The figure shows three views and two pictorial views of one solid part (mm, origin at its lowest corner). Answer the questions. A direction names the side the tool comes from. Coordinates: 2 decimals unless noted, no trailing zeros. Write each loop counter-clockwise with the first axis right and the second up, starting at its lowest first coordinate (ties: lowest second). Pieces come first, ordered by that corner, then holes. Notation, with made-up numbers: M -37,87.25 L -28,87.25 A15 cw -28,100.25 Z; hole C -22,9.25 d8. An arc over 180 degrees is marked long. Write item = value, one per line.
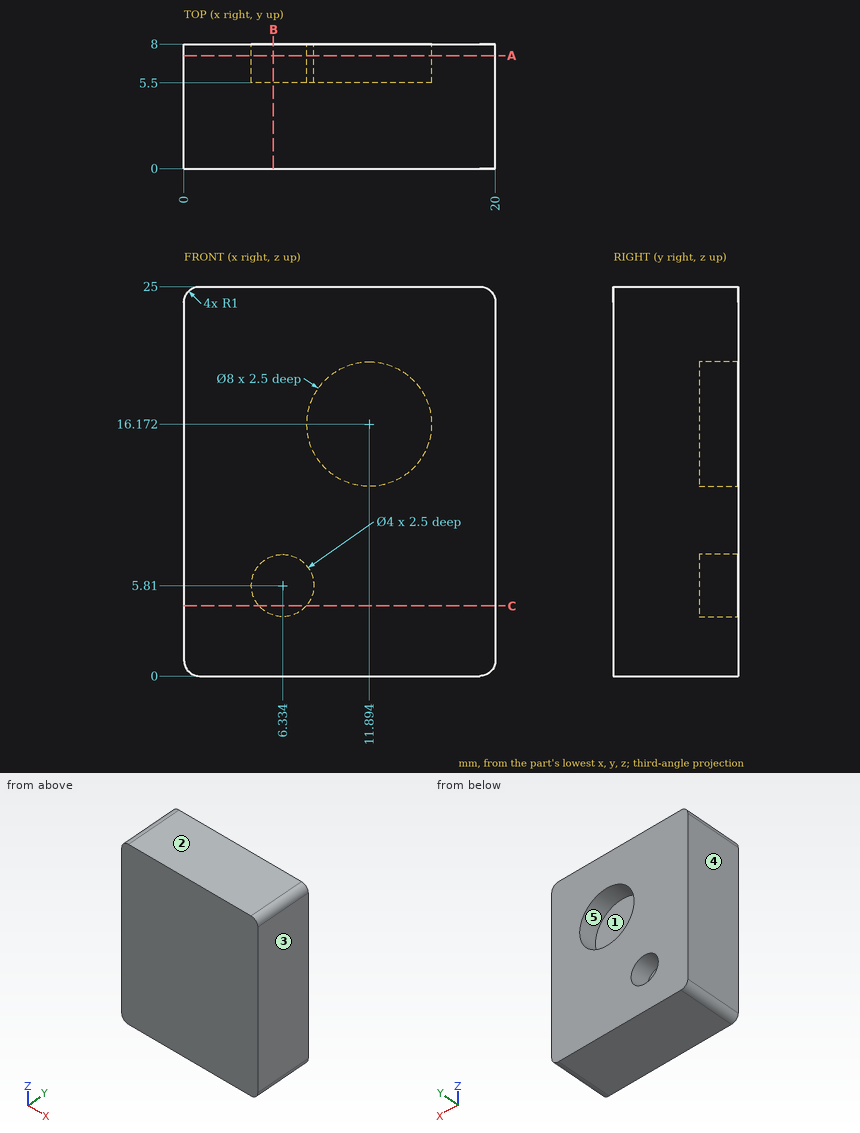
Item 1: Find section A-A (y = 7.25). Determine the outline of the cut face in (x, z), and give its area (3 significant figures).
Worked answers:
outline = M 0,1 A1 ccw 1,0 L 19,0 A1 ccw 20,1 L 20,24 A1 ccw 19,25 L 1,25 A1 ccw 0,24 Z; hole C 6.33,5.81 d4; hole C 11.89,16.17 d8
area = 436 mm²
Item 2: Find section C-C (z = 4.5). Determine the outline of the cut face in (x, y) (1 decimal).
Worked answers:
outline = M 0,0 L 20,0 L 20,8 L 7.8,8 L 7.8,5.5 L 4.8,5.5 L 4.8,8 L 0,8 Z
Item 3: Find section B-B (x = 5.75). Determine the outline of the cut face in (y, z).
Worked answers:
outline = M 0,0 L 8,0 L 8,3.9 L 5.5,3.9 L 5.5,7.72 L 8,7.72 L 8,25 L 0,25 Z
Item 4: Consider line 1 along X through (y, z) = (7, 17.5); line 2 along Z through (x, y) = (13.5, 7.75) (1 decimal); line 3 along Y through (x, z) = (12.25, 18.75). Determine where each line is inside the solid, lowest interval first. Write a range as from..to.
Worked answers:
line_1 = 0..8.12, 15.67..20
line_2 = 0..12.5, 19.8..25
line_3 = 0..5.5
Item 5: Which of the six approach directions +Z, -Z, +X, -X, +Y, -Y give full straight-line access (tool end or side, diameter ignored) to the marked faces 1 and 2?
Worked answers:
face_1 = +Y
face_2 = +Z, +X, -X, +Y, -Y
Item 6: A flat-ended cylindrical pin translates along its axis: pin 1 (5 mm diameter, centred on x = 11.89, z = 16.17, fed in from +Y). Find the tip coordinate at first contact, or state that the pin passes through.
Worked answers:
pin_1 = 5.5
Item 7: For a pull along X with two mould halves and no side action, classify the marked faces 3, 4 and 5 as released by +X, released by -X, zero draft, split by the parting line, or undercut.
Worked answers:
face_3 = released by +X
face_4 = released by -X
face_5 = undercut
